from build123d import *

# Parameters (mm, degrees)
F0_W     = 30
F0_H     = 20
F1_DEPTH = 15
F2_SIZE  = 6


with BuildPart() as f1:
    # F0 (on Top) → F1 (new body)
    with BuildSketch(Plane.XY):
        with Locations((-30, 35)):
            Rectangle(F0_W, F0_H)
        Polygon((45, -25), (45, 25), (15, 25), (-15, 25), (-45, 25), (-45, -25), (-15, -25), (15, -25), align=None)
        with Locations((30, 35)):
            Rectangle(F0_W, F0_H)
        with Locations((30, -35)):
            Rectangle(F0_W, F0_H)
        with Locations((-30, -35)):
            Rectangle(F0_W, F0_H)
    extrude(amount=F1_DEPTH)

    # F2
    f2_edges = [f1.edges().sort_by_distance(p)[0] for p in [
        (-15, 35, 15),
        (-30, 45, 15),
        (-45, 0, 15),
        (-30, -45, 15),
        (-15, -35, 15),
        (0, -25, 15),
        (15, -35, 15),
        (30, -45, 15),
        (45, 0, 15),
        (30, 45, 15),
        (15, 35, 15),
        (0, 25, 15),
        (-15, 35, 0),
        (-30, 45, 0),
        (-45, 0, 0),
        (-30, -45, 0),
        (-15, -35, 0),
        (0, -25, 0),
        (15, -35, 0),
        (30, -45, 0),
        (45, 0, 0),
        (30, 45, 0),
        (15, 35, 0),
        (0, 25, 0),
    ]]
    chamfer(f2_edges, length=F2_SIZE)


solid = f1.part
Part model, mm, in its own coordinate system. A direction names the side the tool comes from. Give positions to 0.01 mm unless a question says otherwise; leave off trailing zeros. Order: outer loops, then holes, each group sorted by start corner. A loop starts at its lowest first (then second) coordinate and runs counter-clockwise, first axis right, second up. Notation, with made-up numbers: (-30, 6) - (5, 6) arc R13 ccw to (5, 12) - close; hole circle Ø11 at (10, -24). An arc over 180 degrees is marked (long way). Use a Markdown table: item, result.
1) 3-axis set-ups, long thin cutter, end or side, ignore diameter. For faces 5 (the flat face through (0, -22, 12)), 6 (the flat face through (0, -22, 3)), 7 (the flat face through (0, 25, 7)), 8 (the flat face through (18, 32, 12)): which of +Z, -Z, +X, -X, +Y, -Y reach the whole face in a straight line?
Checked values:
| item | result |
|---|---|
| face 5 | +Z, -Y |
| face 6 | -Z, -Y |
| face 7 | +Z, -Z, +Y |
| face 8 | +Z, +Y |
2) Saw through at D-D on y = -12.5. List the corners of the cut face in (x, z).
Checked values:
| item | result |
|---|---|
| outline | (-45, 6) - (-39, 0) - (39, 0) - (45, 6) - (45, 9) - (39, 15) - (-39, 15) - (-45, 9) - close |
3) Probe L1, parallel to X at y = -27, z = 6; L2, parallel to Y at x = 3.5, z = 8.75; L3, parallel to X at y = -27, z = 10.25. List the from-to ranges inside material, lowest first. Write a range as from..to.
Checked values:
| item | result |
|---|---|
| L1 | -45..-15, 15..45 |
| L2 | -25..25 |
| L3 | -43.75..-16.25, 16.25..43.75 |
4) Flat gauge pins, fed straight in: P1, Ø1.5, axis at x = -3, z = 6.5, coming from the -Y side; P2, Ø4, axis at x = 16, y = -32.5, coming from the -Z side; P3, Ø5, axis at x = 8, z = 8, coming from the +Y side. Where does each tip first touch, or does it go through?
Checked values:
| item | result |
|---|---|
| P1 | y = -25 |
| P2 | z = 3 |
| P3 | y = 25 |
5) Saw through at A-A on y = -27.5. List the corners of the cut face in (x, z).
Checked values:
| item | result |
|---|---|
| outline | (-45, 6) - (-39, 0) - (-21, 0) - (-15, 6) - (-15, 9) - (-21, 15) - (-39, 15) - (-45, 9) - close; (15, 6) - (21, 0) - (39, 0) - (45, 6) - (45, 9) - (39, 15) - (21, 15) - (15, 9) - close |
6) Two-plate mould, pull along X, no slides. Class faces 1 (the flat face through (15, 35, 7)), 2 (the flat face through (-45, 1, 7)), 3 (the flat face through (30, 42, 3)), 4 (the flat face through (18, -32, 12)): +X half, -X half, draft (parallel to the pull), parting line (faces both ways), or undercut.
Checked values:
| item | result |
|---|---|
| face 1 | undercut |
| face 2 | -X half |
| face 3 | draft |
| face 4 | undercut |
7) Saw through at C-C on z = 10.25. List the corners of the cut face in (x, y), plus the area to 3 significant figures.
Checked values:
| item | result |
|---|---|
| outline | (-43.75, -43.75) - (-16.25, -43.75) - (-16.25, -23.75) - (16.25, -23.75) - (16.25, -43.75) - (43.75, -43.75) - (43.75, 43.75) - (16.25, 43.75) - (16.25, 23.75) - (-16.25, 23.75) - (-16.25, 43.75) - (-43.75, 43.75) - close |
| area | 6,360 mm² |
8) Saw through at B-B on x = 19. List the corners of the cut face in (y, z), plus the area to 3 significant figures.
Checked values:
| item | result |
|---|---|
| outline | (-45, 6) - (-41, 2) - (-21, 2) - (-19, 0) - (19, 0) - (21, 2) - (41, 2) - (45, 6) - (45, 9) - (41, 13) - (21, 13) - (19, 15) - (-19, 15) - (-21, 13) - (-41, 13) - (-45, 9) - close |
| area | 1,120 mm² |
